Model file for the job. Use its own axes, mm. Face numbers are marked on the shaded views. A direction names the side the tool comes from. Give positions to 0.01 mm unless a question says otherwise; leave off trailing zeros. Order: outer loops, then holes, each group sorted by start corner. A loop starts at its lowest first (then second) coordinate and runs counter-clockwise, first axis right, second up. Notation, with made-up numbers: M 50.5,0 L 57.5,0 A20 ccw 57.5,32 Z; hole C 29.25,28 d6. An arc over 180 degrees is marked long. Return JSON: item names as keys, results as strings. Group by question number.
1. Wall check: probe 1 along Z at (x, y) = (3, -52); probe 2 along Z at (x, y) = (3, 50); probe 3 along Z at (x, y) = (3, 44). Give the ranges that are in metal, low to high. Write a range as [from, to].
2. Pin check, flat tips, straight feed: pin 1 (3 mm diameter, centred on x = 20.5, y = -28, fed in from -Z); pin 2 (12 mm diameter, centred on x = -42.5, z = 53.5, fed in from -Y); pin 3 (23.5 mm diameter, centred on x = 8, y = -13, fed in from +Z); pin 4 (16 mm diameter, centred on x = 3, z = 26, fed in from +Y). Stop position of each tip, or through.
3. Two-plate mould, pull along Y, no slides. Class the marked faces 1, 2 and 3: released by +Y, released by -Y, zero draft, split by the parting line, or undercut.
4. Slice it at B-B on y = -42. Give the number of separate pieces and of enclosed holes in the cut face, then the cut area to 3 significant figures.
5. 3-axis set-ups, long thin cutter, end or side, ignore diameter. For the marked faces 4 and 5: which of +Z, -Z, +X, -X, +Y, -Y reach the whole face in a straight line?
6. Slice it at A-A on z = 26. List the corners of the cut face in (x, y), then the cut area to 3 significant figures.
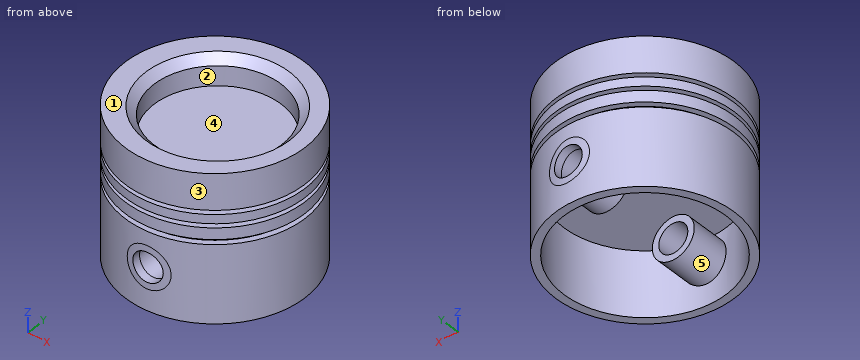
from build123d import *

# Parameters (mm, degrees)
F0_R           = 55
F1_DEPTH       = 47.5
F2_R           = 51.5
F3_DEPTH       = 3
F4_R           = 55
F5_DEPTH       = 7
F6_R           = 51.5
F7_DEPTH       = 2.5
F8_R           = 55
F9_DEPTH       = 5.5
F10_R          = 51.5
F11_DEPTH      = 2.5
F12_R          = 55
F12_R_2        = 39
F13_DEPTH      = 22
F14_R          = 50
F15_DEPTH      = 40
F16_R          = 43.5007627275
F17_DEPTH      = 5
F18_SIZE       = 5
F19_R          = 13
F19_R_2        = 9
F20_DEPTH      = 62
F20_DEPTH_BACK = 70.1
F21_R          = 9
F22_DEPTH      = 75.8
F22_DEPTH_BACK = 99.3
F24_DEPTH      = 40
F25_R          = 82.1696032424
F25_R_2        = 55
F26_DEPTH      = 32.2


with BuildPart() as f1:
    # F0 (on Top) → F1 (new body)
    with BuildSketch(Plane.XY):
        Circle(F0_R)
    extrude(amount=F1_DEPTH)

    # F2 (on face) → F3 (join)
    with BuildSketch(Plane.XY.offset(47.5)):
        Circle(F2_R)
    extrude(amount=F3_DEPTH)

    # F4 (on face) → F5 (join)
    with BuildSketch(Plane.XY.offset(50.5)):
        Circle(F4_R)
    extrude(amount=F5_DEPTH)

    # F6 (on face) → F7 (join)
    with BuildSketch(Plane.XY.offset(57.5)):
        Circle(F6_R)
    extrude(amount=F7_DEPTH)

    # F8 (on face) → F9 (join)
    with BuildSketch(Plane.XY.offset(60)):
        Circle(F8_R)
    extrude(amount=F9_DEPTH)

    # F10 (on face) → F11 (join)
    with BuildSketch(Plane.XY.offset(65.5)):
        Circle(F10_R)
    extrude(amount=F11_DEPTH)

    # F12 (on face) → F13 (join)
    with BuildSketch(Plane.XY.offset(68)):
        Circle(F12_R)
        with Locations((1.679461333, 0)):
            Circle(F12_R_2, mode=Mode.SUBTRACT)
    extrude(amount=F13_DEPTH)

    # F14 (on face) → F15 (cut)
    with BuildSketch(Plane(origin=(0, 0, 0), x_dir=(1, 0, 0), z_dir=(0, 0, -1))):
        Circle(F14_R)
    extrude(amount=-F15_DEPTH, mode=Mode.SUBTRACT)

    # F16 (on face) → F17 (join)
    with BuildSketch(Plane.XY.offset(68)):
        Circle(F16_R)
    extrude(amount=F17_DEPTH)

    # F18
    f18_edges = [f1.edges().sort_by_distance(p)[0] for p in [
        (-37.320539, 0, 90),
    ]]
    chamfer(f18_edges, length=F18_SIZE)

    # F19 (on Front) → F20 (join, two sides)
    with BuildSketch(Plane.XZ) as f20_sk:
        with Locations((3, 26)):
            Circle(F19_R)
        with Locations((3, 26)):
            Circle(F19_R_2, mode=Mode.SUBTRACT)
    extrude(amount=F20_DEPTH)
    extrude(f20_sk.sketch, amount=-F20_DEPTH_BACK)

    # F21 (on Front) → F22 (cut, two sides)
    with BuildSketch(Plane.XZ) as f22_sk:
        with Locations((3, 26)):
            Circle(F21_R)
    extrude(amount=-F22_DEPTH, mode=Mode.SUBTRACT)
    extrude(f22_sk.sketch, amount=F22_DEPTH_BACK, mode=Mode.SUBTRACT)

    # F23 (on Top) → F24 (cut)
    with BuildSketch(Plane.XY):
        with BuildLine():
            Line((-10, 25), (-10, 48.9897948557))
            ThreePointArc((-10, 48.9897948557), (-50, 0), (-10, -48.9897948557))
            Line((-10, -48.9897948557), (-10, -25))
            Line((-10, -25), (16, -25))
            Line((16, -25), (16, -47.3708771293))
            ThreePointArc((16, -47.3708771293), (50, 0), (16, 47.3708771293))
            Line((16, 47.3708771293), (16, 25))
            Line((16, 25), (-10, 25))
        make_face()
    extrude(amount=F24_DEPTH, mode=Mode.SUBTRACT)

    # F25 (on face) → F26 (cut)
    with BuildSketch(Plane(origin=(0, 0, 40), x_dir=(1, 0, 0), z_dir=(0, 0, -1))):
        with Locations((0, -2.1747821011)):
            Circle(F25_R)
        Circle(F25_R_2, mode=Mode.SUBTRACT)
    extrude(amount=F26_DEPTH, mode=Mode.SUBTRACT)


solid = f1.part
Result:
{
 "1": {"probe 1": "z = [0, 17], [35, 47.5], [50.5, 57.5], [60, 65.5], [68, 90]", "probe 2": "z = [0, 17], [35, 90]", "probe 3": "z = [13, 17], [35, 39], [40, 90]"},
 "2": {"pin 1": "stops at z = 40", "pin 2": "stops at y = -41.14", "pin 3": "stops at z = 73", "pin 4": "passes through"},
 "3": {"face 1": "zero draft", "face 2": "undercut", "face 3": "split by the parting line"},
 "4": {"separate pieces": "2", "enclosed holes": "1", "area": "4,370 mm2"},
 "5": {"face 4": "+Z", "face 5": "none"},
 "6": {"outline": "M -10,-48.99 A50 cw -10,48.99 L -10,25 L -6,25 L -6,54.67 A55 ccw -6,-54.67 L -6,-25 L -10,-25 Z; M 12,-53.67 A55 ccw 12,53.67 L 12,25 L 16,25 L 16,47.37 A50 cw 16,-47.37 L 16,-25 L 12,-25 Z", "area": "1,850 mm2"}
}
